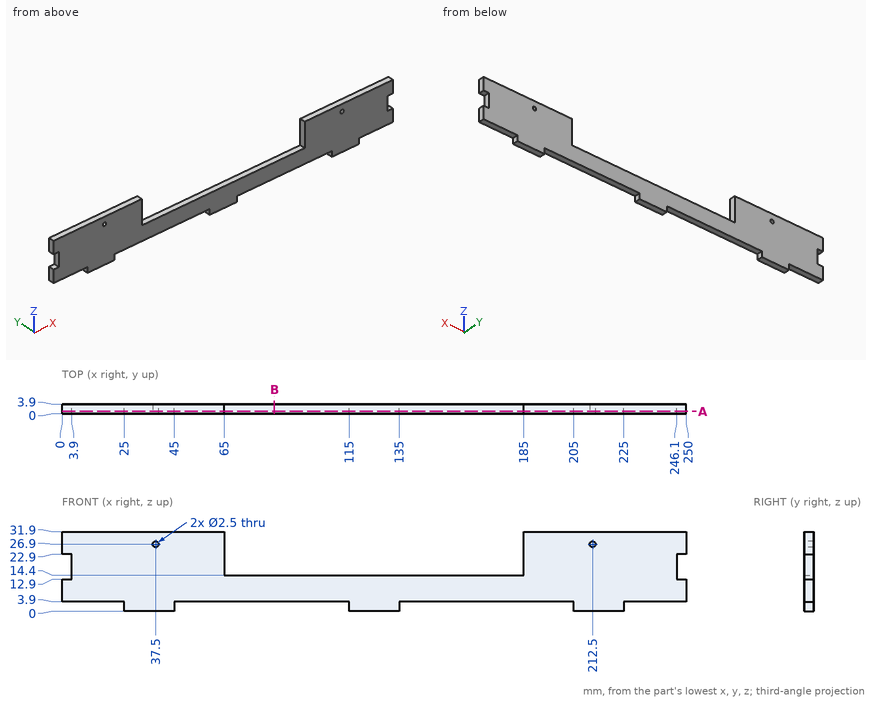
Can you work these out from the drawing? Everything is in mm from the part's minimum corner. Round coordinates to 2 decimals unless told otherwise and drop trailing zeros. Loops run counter-clockwise (first coordinate to the right, second up) from the corner with the lowest first, then second, coordinate; pieces in that order, holes last. Notation, with made-up numbers: M 13,56.5 L 60,56.5 A11 ccw 60,63.5 Z; hole C 21,72 d4. An arc over 180 degrees is marked long. Write item = value, one per line.
1. I need wall thicknesses on probe 1 along X at (y, z) = (1.2, 26.9); probe 2 along Z at (x, y) = (37.5, 2.25); probe 3 along X at (y, z) = (3.55, 22). Which ranges of each line are inside material? Lowest first, please.
Results below:
probe_1 = 0 to 36.25, 38.75 to 65, 185 to 211.25, 213.75 to 250
probe_2 = 0 to 25.65, 28.15 to 31.9
probe_3 = 3.9 to 65, 185 to 246.1
2. I want a section at B-B, the plane x = 85. Write out the boundary of the cut face in (y, z).
Results below:
outline = M 0,3.9 L 3.9,3.9 L 3.9,14.4 L 0,14.4 Z
3. Will these pins go through, and if not, where does the flat tip stop? P1, Ø1.9, axis at y = 1.5, z = 2.5, coming from the +X side; P2, Ø1.5, axis at x = 59.5, y = 1, coming from the -Z side; P3, Ø1.2, axis at y = 3, z = 2.5, coming from the -X side.
Results below:
P1 = 225
P2 = 3.9
P3 = 25
4. I want a section at A-A, the plane y = 0.95. Count the separate pieces of the cut face and the enclosed holes in it, and give its area (3 significant figures).
Results below:
separate_pieces = 1
enclosed_holes = 2
area = 5,050 mm²
